Could you check a few things on this model? Use its own coordinates, in mm. Face numbers are marked on the shaded views. A direction names the side the tool comes from. Coordinates: 2 decimals unless noted, no trailing zeros. Answer as CSV lines item,"result". Start each with the question number.
Item 1: On a 3-axis mill with a long thin cutter (end or side, diameter ignored), from which of +Z, -Z, +X, -X, +Y, -Y can I reach the whole of each face in a straight line? I mean the marked faces 3, 4 and 5. Say none if no direction works.
Item 2: Suppose I cut it at A-A, the plane x = -22.5. State how many separate pieces and enclosed holes the cut face has, and give its area (3 significant figures).
Item 3: We'd pull the mould along X, two halves only. Please class the marked faces 1 and 2: +X half, -X half, draft (parallel to the pull), parting line (faces both ways), or undercut.
Item 4: If I drill on line 1 along Z through (x, y) = (12.5, -0.45); line 2 along Z through (x, y) = (22.5, -5.55); line 3 along X through (y, z) = (-4.2, -13.5), over which ranges is the centre line in solid material (lowest first)? Write a range as [from, to].
Item 5: I'm going to push flat-ended pins straight in: P1, Ø1.5, axis at x = 18, y = -0.5, coming from the +Z side; P2, Ø2, axis at y = -3.5, z = -8, coming from the +X side; P3, Ø2, axis at x = 6.5, z = -5.5, coming from the -Y side; P4, Ø3, axis at x = 22.5, z = -15, coming from the -Y side. Where does each tip first touch, or does it pass through?
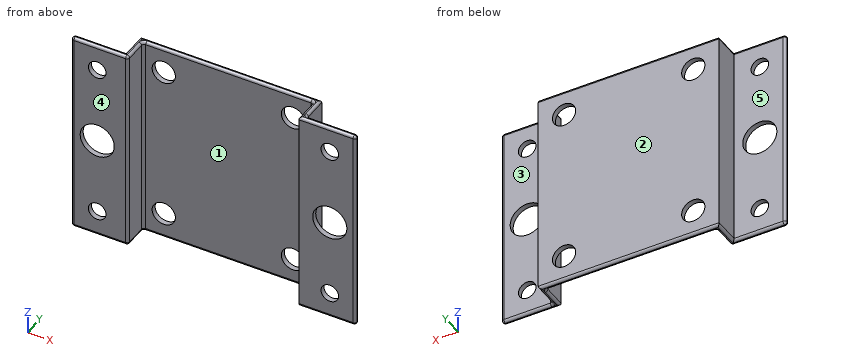
```python
from build123d import *

# Parameters (mm, degrees)
BOSS_EXTRUDE1_DEPTH  = 20
FILLET1_R            = 0.5
M6_CLEARANCE_HOLE1_D = 6.6
M4_CLEARANCE_HOLE1_D = 4.5
M3_CLEARANCE_HOLE1_D = 3.4
MIRROR2_COPY_1_D     = 4.5
MIRROR2_COPY_2_D     = 3.4


with BuildPart() as part:
    # Sketch1 → Boss-Extrude1 (new, symmetric)
    with BuildSketch(Plane.XY):
        Polygon((-17.5, 0), (17.5, 0), (17.5, -5), (27.5, -5), (27.5, -6), (16.5, -6), (16.5, -1), (-16.5, -1), (-16.5, -6), (-27.5, -6), (-27.5, -5), (-17.5, -5), align=None)
    extrude(amount=BOSS_EXTRUDE1_DEPTH, both=True)

    # Fillet1
    fillet1_edges = [part.edges().sort_by_distance(p)[0] for p in [
        (27.5, -5.5, -20),
        (22, -6, -20),
        (0, 0, 20),
        (16.5, -3.5, -20),
        (0, -1, -20),
        (-16.5, -3.5, -20),
        (-22, -6, -20),
        (-27.5, -5.5, -20),
        (-22.5, -5, -20),
        (-17.5, -2.5, -20),
        (0, 0, -20),
        (17.5, -2.5, -20),
        (22.5, -5, -20),
        (-17.5, -2.5, 20),
        (27.5, -5, 0),
        (27.5, -6, 0),
        (-22.5, -5, 20),
        (16.5, -1, 0),
        (-16.5, -1, 0),
        (-16.5, -6, 0),
        (-27.5, -6, 0),
        (-27.5, -5, 0),
        (17.5, -5, 0),
        (-27.5, -5.5, 20),
        (-22, -6, 20),
        (-16.5, -3.5, 20),
        (0, -1, 20),
        (16.5, -3.5, 20),
        (22, -6, 20),
        (27.5, -5.5, 20),
        (22.5, -5, 20),
        (17.5, -2.5, 20),
    ]]
    fillet(fillet1_edges, radius=FILLET1_R - 0.0001)  # a hair under: the kernel refuses the full size

    # M6 Clearance Hole1 (through all)
    with Locations(Plane(origin=(0, -5, 0), x_dir=(1, 0, 0), z_dir=(0, 1, 0))):
        with Locations((-22.5, 0), (22.5, 0)):
            Hole(M6_CLEARANCE_HOLE1_D / 2)

    # M4 Clearance Hole1 (through all)
    with Locations(Plane(origin=(0, 0, 0), x_dir=(1, 0, 0), z_dir=(0, 1, 0))):
        with Locations((-12.5, 15)):
            m4_clearance_hole1 = Hole(M4_CLEARANCE_HOLE1_D / 2)

    # M3 Clearance Hole1 (through all)
    with Locations(Plane(origin=(0, -5, 0), x_dir=(1, 0, 0), z_dir=(0, 1, 0))):
        with Locations((-22.5, 15)):
            m3_clearance_hole1 = Hole(M3_CLEARANCE_HOLE1_D / 2)

    # Mirror1: M4 Clearance Hole1, M3 Clearance Hole1 across plane
    add(m4_clearance_hole1.mirror(Plane(origin=(0, 0, 0), x_dir=(0, 0, 1), z_dir=(1, 0, 0))), mode=Mode.SUBTRACT)
    add(m3_clearance_hole1.mirror(Plane(origin=(0, 0, 0), x_dir=(0, 0, 1), z_dir=(1, 0, 0))), mode=Mode.SUBTRACT)

    # Mirror2: M4 Clearance Hole1, M3 Clearance Hole1 across plane
    add(m4_clearance_hole1.mirror(Plane.XY), mode=Mode.SUBTRACT)
    add(m3_clearance_hole1.mirror(Plane.XY), mode=Mode.SUBTRACT)

    # Mirror2 copy 1 (through all)
    with Locations(Plane(origin=(0, 0, 0), x_dir=(-1, 0, 0), z_dir=(0, 1, 0))):
        with Locations((-12.5, 15)):
            Hole(MIRROR2_COPY_1_D / 2)

    # Mirror2 copy 2 (through all)
    with Locations(Plane(origin=(0, -5, 0), x_dir=(-1, 0, 0), z_dir=(0, 1, 0))):
        with Locations((-22.5, 15)):
            Hole(MIRROR2_COPY_2_D / 2)


solid = part.part
```
Ans:
1,face 3,"+Z, -Z, +X, +Y"
1,face 4,"+Z, -Z, +X, -X, -Y"
1,face 5,"+Z, -Z, -X, +Y"
2,separate pieces,"4"
2,enclosed holes,"0"
2,area,"26.4 mm^2"
3,face 1,"undercut"
3,face 2,"draft"
4,line 1,"z = [-20, -17.25], [-12.75, 12.75], [17.25, 20]"
4,line 2,"z = [-20, -16.7], [-13.3, -3.3], [3.3, 13.3], [16.7, 20]"
4,line 3,"x = [-17.5, -16.5], [16.5, 17.5]"
5,P1,"stops at z = 19.93"
5,P2,"stops at x = 17.5"
5,P3,"stops at y = -1"
5,P4,"passes through"
